Here's how the part is built. I have some questions about the finished solid (model axes, mm). Face numbers are marked on the shaded views. Give positions to 0.01 mm unless a question says otherwise; leave off trailing zeros. Order: outer loops, then holes, each group sorted by start corner. A loop starts at its lowest first (then second) coordinate and runs counter-clockwise, first axis right, second up.
from build123d import *

# Parameters (mm, degrees)
EXTRUDE_1_DEPTH     = 4
SKETCH_2_W          = 15
SKETCH_2_H          = 13.3866
CUT_EXTRUDE_1_DEPTH = 121.93395925
SKETCH_3_W          = 10
SKETCH_3_H          = 10
SKETCH_3_R          = 1.55
SKETCH_3_H_2        = 14.755
EXTRUDE_2_DEPTH     = 4
EXTRUDE_3_DEPTH     = 4
EXTRUDE_4_DEPTH     = 4
SKETCH_7_W          = 27.8
SKETCH_7_H          = 4
EXTRUDE_5_DEPTH     = 4
EXTRUDE_START       = -4
EXTRUDE_6_DEPTH     = 4
SKETCH_11_W         = 16.8
SKETCH_11_H         = 10.85
CUT_EXTRUDE_2_DEPTH = 133.52791749
CHAMFER_1_SIZE      = 2
CHAMFER_2_SIZE      = 2
SKETCH_12_W         = 12
SKETCH_12_H         = 8.55
SKETCH_12_R         = 1.25
EXTRUDE_7_DEPTH     = 4
EXTRUDE_START_2     = 4
SKETCH_13_R         = 1.25
SKETCH_13_W         = 4
SKETCH_13_H         = 8.709663749
EXTRUDE_8_DEPTH     = 4
SKETCH_14_R         = 1
CUT_EXTRUDE_3_DEPTH = 132.839329922
SKETCH_15_R         = 0.9
EXTRUDE_9_DEPTH     = 1
FILLET_1_R          = 0.9
CUT_EXTRUDE_START   = -1.7
SKETCH_16_R         = 1
CUT_EXTRUDE_4_DEPTH = 1.7
CUT_EXTRUDE_5_DEPTH = 132.839329922
SKETCH_19_W         = 5
SKETCH_19_H         = 38.5268
SKETCH_19_W_2       = 8.236887868
SKETCH_19_H_2       = 1.55
CUT_EXTRUDE_6_DEPTH = 132.839329922
EXTRUDE_12_DEPTH    = 23.28
CUT_EXTRUDE_7_REACH = 100.821
SKETCH_23_R         = 1.55
EXTRUDE_13_DEPTH    = 4
CUT_EXTRUDE_START_2 = -19.28
CUT_EXTRUDE_8_DEPTH = 19.48
SKETCH_26_W         = 10.1
SKETCH_26_H         = 2
EXTRUDE_14_DEPTH    = 3


# Read off the part's stored shape, not the designer's step: the extrude step
with BuildPart() as part:
    # Sketch 1 → Extrude 1 (new body)
    with BuildSketch(Plane.XY):
        with BuildLine():
            Line((-16.4, -7.25), (-16.4, 119.75))
            Line((-16.4, 119.75), (16.4, 119.75))
            Line((16.4, 119.75), (16.4, -7.25))
            ThreePointArc((16.4, -7.25), (15.038046533, -10.538046533), (11.75, -11.9))
            Line((11.75, -11.9), (-11.75, -11.9))
            ThreePointArc((-11.75, -11.9), (-15.038046533, -10.538046533), (-16.4, -7.25))
        make_face()
    extrude(amount=EXTRUDE_1_DEPTH)

    # Sketch 2 → Cut-Extrude 1 (cut, through all)
    with BuildSketch(Plane(origin=(0, 0, 0), x_dir=(-1, 0, 0), z_dir=(0, 0, -1))):
        with Locations((0, 110.2067)):
            Rectangle(SKETCH_2_W, SKETCH_2_H)
    extrude(amount=-CUT_EXTRUDE_1_DEPTH, mode=Mode.SUBTRACT)

    # Sketch 3 → Extrude 2 (add)
    # profile 1 of 2: a face of its own
    with BuildSketch(Plane(origin=(0, 119.75, 0), x_dir=(1, 0, 0), z_dir=(0, 1, 0))):
        with Locations((-18.9, 15.755)):
            Rectangle(SKETCH_3_W, SKETCH_3_H)
        with Locations(Location((-18.9, 15.755, 0), (0, 0, 270))):
            Circle(SKETCH_3_R, mode=Mode.SUBTRACT)
    # profile 2 of 2: a face of its own
    with BuildSketch(Plane(origin=(0, 119.75, 0), x_dir=(1, 0, 0), z_dir=(0, 1, 0))):
        with Locations((-18.9, 3.3775)):
            Rectangle(SKETCH_3_W, SKETCH_3_H_2)
    extrude_2 = extrude(amount=-EXTRUDE_2_DEPTH)

    # Mirror 1: Extrude 2 across plane
    add(extrude_2.mirror(Plane(origin=(0, 0, 0), x_dir=(0, 0, 1), z_dir=(1, 0, 0))))

    # Sketch 6 → Extrude 4 (add)
    with BuildSketch(Plane.XY.offset(4)):
        Polygon((-16.4, 115.75), (-23.9, 115.75), (-16.4, 108.25), align=None)
        Polygon((16.4, 115.75), (16.4, 108.25), (23.9, 115.75), align=None)
    extrude(amount=-EXTRUDE_4_DEPTH)

    # Sketch 7 → Extrude 5 (add)
    with BuildSketch(Plane(origin=(0, 119.75, 0), x_dir=(1, 0, 0), z_dir=(0, 1, 0))):
        with Locations((0, 18.755)):
            Rectangle(SKETCH_7_W, SKETCH_7_H)
    extrude(amount=-EXTRUDE_5_DEPTH)



with BuildPart() as body_2:
    # Sketch 5 → Extrude 3 (new body)
    with BuildSketch(Plane(origin=(0, 2.890336251, 0), x_dir=(1, 0, 0), z_dir=(0, 1, 0))):
        Polygon((50.795757056, 9.855), (46.095757056, 9.855), (32.240757056, -4), (39.311824868, -4), (51.095757056, 7.783932188), (51.095757056, 9.855), align=None)
        with BuildLine():
            Line((50.795757056, 18.755), (46.095757056, 18.755))
            Line((46.095757056, 18.755), (46.095757056, 9.855))
            Line((46.095757056, 9.855), (50.795757056, 9.855))
            Line((50.795757056, 9.855), (50.795757056, 15.105))
            Line((50.795757056, 15.105), (49.255691264, 15.105))
            ThreePointArc((49.255691264, 15.105), (47.495757056, 15.755), (49.255691264, 16.405))
            Line((49.255691264, 16.405), (50.795757056, 16.405))
            Line((50.795757056, 16.405), (50.795757056, 18.755))
        make_face()
        with BuildLine():
            Line((51.095757056, 18.755), (50.795757056, 18.755))
            Line((50.795757056, 18.755), (50.795757056, 16.405))
            Line((50.795757056, 16.405), (49.255691264, 16.405))
            ThreePointArc((49.255691264, 16.405), (49.433822674, 16.10145764), (49.495757056, 15.755))
            ThreePointArc((49.495757056, 15.755), (49.433822674, 15.40854236), (49.255691264, 15.105))
            Line((49.255691264, 15.105), (50.795757056, 15.105))
            Line((50.795757056, 15.105), (50.795757056, 9.855))
            Line((50.795757056, 9.855), (51.095757056, 9.855))
            Line((51.095757056, 9.855), (51.095757056, 18.755))
        make_face()
    extrude(amount=EXTRUDE_3_DEPTH)


with BuildPart() as part_1:
    add(part.part)

    add(body_2.part)  # Extrude 6 merges body 2
    # Sketch 8 → Extrude 6 (add)
    with BuildSketch(Plane.XY.offset(4).offset(EXTRUDE_START)):
        with BuildLine():
            Line((26.521488617, -11.9), (39.311824868, 0.890336251))
            Line((39.311824868, 0.890336251), (39.311824868, 6.890336251))
            Line((39.311824868, 6.890336251), (16.4, 6.890336251))
            Line((16.4, 6.890336251), (16.4, -7.25))
            ThreePointArc((16.4, -7.25), (15.038046533, -10.538046533), (11.75, -11.9))
            Line((11.75, -11.9), (26.521488617, -11.9))
        make_face()
    extrude(amount=EXTRUDE_6_DEPTH)

    # Sketch 11 → Cut-Extrude 2 (cut, through all)
    with BuildSketch(Plane.XY.offset(4)):
        with Locations((0, 1.525)):
            Rectangle(SKETCH_11_W, SKETCH_11_H)
        with Locations((0, 22.975)):
            Rectangle(SKETCH_11_W, SKETCH_11_H)
    extrude(amount=-CUT_EXTRUDE_2_DEPTH, mode=Mode.SUBTRACT)

    # Chamfer 1
    chamfer_1_edges = [part_1.edges().sort_by_distance(p)[0] for p in [
        (39.311824868, 2.890336251, 2),
    ]]
    chamfer(chamfer_1_edges, length=CHAMFER_1_SIZE - 0.0001)  # a hair under: the kernel refuses the full size

    # Chamfer 2
    chamfer_2_edges = [part_1.edges().sort_by_distance(p)[0] for p in [
        (38.776240962, 2.890336251, 0),
    ]]
    chamfer(chamfer_2_edges, length=CHAMFER_2_SIZE - 0.0001)  # a hair under: the kernel refuses the full size

    # Sketch 12 → Extrude 7 (add)
    with BuildSketch(Plane.ZY.offset(16.4)):
        with Locations((-2, 13.325)):
            Rectangle(SKETCH_12_W, SKETCH_12_H)
        with Locations((-4, 12.25)):
            Circle(SKETCH_12_R, mode=Mode.SUBTRACT)
    extrude(amount=EXTRUDE_7_DEPTH)

    # Sketch 13 → Extrude 8 (add)
    # profile 1 of 2: a face of its own
    with BuildSketch(Plane(origin=(16.4, 0, 0), x_dir=(0, 0, -1), z_dir=(1, 0, 0)).offset(EXTRUDE_START_2)):
        Polygon((8, 9.890336251), (8, 15.6), (0, 15.6), (0, 6.890336251), (5, 6.890336251), align=None)
        with Locations(Location((4, 12.25, 0), (0, 0, 180))):
            Circle(SKETCH_13_R, mode=Mode.SUBTRACT)
    # profile 2 of 2: a face of its own
    with BuildSketch(Plane(origin=(16.4, 0, 0), x_dir=(0, 0, -1), z_dir=(1, 0, 0)).offset(EXTRUDE_START_2)):
        with Locations((-2, 11.245168126)):
            Rectangle(SKETCH_13_W, SKETCH_13_H)
    extrude(amount=-EXTRUDE_8_DEPTH)

    # Sketch 14 → Cut-Extrude 3 (cut, through all)
    with BuildSketch(Plane(origin=(0, 0, 0), x_dir=(-1, 0, 0), z_dir=(0, 0, -1))):
        with Locations((-5, 62.6)):
            Circle(SKETCH_14_R)
        with Locations((-5, 99)):
            Circle(SKETCH_14_R)
    extrude(amount=-CUT_EXTRUDE_3_DEPTH, mode=Mode.SUBTRACT)

    # Sketch 15 → Extrude 9 (add)
    with BuildSketch(Plane(origin=(0, 0, 0), x_dir=(-1, 0, 0), z_dir=(0, 0, -1))):
        with Locations(Location((-5, 94.35, 0), (0, 0, 180))):
            Circle(SKETCH_15_R)
        with Locations(Location((-5, 57.98, 0), (0, 0, 180))):
            Circle(SKETCH_15_R)
    extrude(amount=EXTRUDE_9_DEPTH)

    # Fillet 1
    fillet_1_edges = [part_1.edges().sort_by_distance(p)[0] for p in [
        (4.1, 94.35, -1),
        (4.1, 57.98, -1),
    ]]
    fillet(fillet_1_edges, radius=FILLET_1_R)

    # Sketch 16 → Cut-Extrude 4 (cut)
    # profile 1 of 2: a face of its own
    with BuildSketch(Plane.XY.offset(4).offset(CUT_EXTRUDE_START)):
        Polygon((7.05, 61.416431948), (7.05, 63.783568052), (5, 64.967136104), (2.95, 63.783568052), (2.95, 61.416431948), (5, 60.232863896), align=None)
        with Locations(Location((5, 62.6, 0), (0, 0, 180))):
            Circle(SKETCH_16_R, mode=Mode.SUBTRACT)
    # profile 2 of 2: a face of its own
    with BuildSketch(Plane.XY.offset(4).offset(CUT_EXTRUDE_START)):
        Polygon((2.95, 97.816431948), (5, 96.632863896), (7.05, 97.816431948), (7.05, 100.183568052), (5, 101.367136104), (2.95, 100.183568052), align=None)
        with Locations(Location((5, 99, 0), (0, 0, 180))):
            Circle(SKETCH_16_R, mode=Mode.SUBTRACT)
    extrude(amount=CUT_EXTRUDE_4_DEPTH, mode=Mode.SUBTRACT)

    # Sketch 17 → Cut-Extrude 5 (cut, symmetric)
    with BuildSketch(Plane(origin=(0, 0, 0), x_dir=(-1, 0, 0), z_dir=(0, 0, -1))):
        Polygon((-12.5, 104.35), (-16.4, 108.25), (-16.4, 40.0866), (-12.5, 43.9866), align=None)
    cut_extrude_5 = extrude(amount=CUT_EXTRUDE_5_DEPTH, both=True, mode=Mode.SUBTRACT)

    # Mirror 2: Cut-Extrude 5 across plane
    add(cut_extrude_5.mirror(Plane(origin=(0, 0, 0), x_dir=(0, 0, 1), z_dir=(1, 0, 0))), mode=Mode.SUBTRACT)

    # Sketch 19 → Cut-Extrude 6 (cut, through all)
    with BuildSketch(Plane(origin=(0, 0, 0), x_dir=(-1, 0, 0), z_dir=(0, 0, -1))):
        with Locations((2, 74.25)):
            Rectangle(SKETCH_19_W, SKETCH_19_H)
        with Locations((0, 47.675)):
            Rectangle(SKETCH_19_W_2, SKETCH_19_H_2)
    extrude(amount=-CUT_EXTRUDE_6_DEPTH, mode=Mode.SUBTRACT)

    # Sketch 22 → Extrude 12 (add)
    with BuildSketch(Plane.XY.offset(4)):
        with BuildLine():
            Line((16.4, 32.719535971), (16.4, 31.75))
            Line((16.4, 31.75), (22.425, 31.75))
            Line((22.425, 31.75), (22.425, 37.75))
            Line((22.425, 37.75), (11.75, 37.75))
            Line((11.75, 37.75), (11.75, 36.5))
            ThreePointArc((11.75, 36.5), (14.746431556, 35.435633993), (16.4, 32.719535971))
        make_face()
    extrude_12 = extrude(amount=-EXTRUDE_12_DEPTH)

    # Sketch 23 → Cut-Extrude 7 (cut, up to next)
    with BuildSketch(Plane(origin=(0, 37.75, 0), x_dir=(1, 0, 0), z_dir=(0, 1, 0)), mode=Mode.PRIVATE) as cut_extrude_7_sk1:
        with Locations(Location((18.9, 15.755, 0), (0, 0, 270))):
            Circle(SKETCH_23_R)
    cut_extrude_7_tool1 = extrude(cut_extrude_7_sk1.sketch, amount=-CUT_EXTRUDE_7_REACH, mode=Mode.PRIVATE) & part_1.part
    # Sketch 23 → Cut-Extrude 7 (cut, up to next)
    with BuildSketch(Plane(origin=(0, 37.75, 0), x_dir=(1, 0, 0), z_dir=(0, 1, 0)), mode=Mode.PRIVATE) as cut_extrude_7_sk2:
        with BuildLine():
            ThreePointArc((18.9, 19.28), (21.392551404, 18.247551403), (22.425, 15.754999999))
            Line((22.425, 15.754999999), (22.425, 19.28))
            Line((22.425, 19.28), (18.9, 19.28))
        make_face()
    cut_extrude_7_tool2 = extrude(cut_extrude_7_sk2.sketch, amount=-CUT_EXTRUDE_7_REACH, mode=Mode.PRIVATE) & part_1.part
    cut_extrude_7_1 = cut_extrude_7_tool1.solids().sort_by_distance((18.9, 37.75, -15.755))[0]
    add(cut_extrude_7_1, mode=Mode.SUBTRACT)
    cut_extrude_7_2 = cut_extrude_7_tool2.solids().sort_by_distance((21.637628, 37.75, -18.492628))[0]
    add(cut_extrude_7_2, mode=Mode.SUBTRACT)
    cut_extrude_7 = cut_extrude_7_1 + cut_extrude_7_2  # Cut-Extrude 7 as one shape, for the pattern or mirror that repeats it

    # Sketch 24 → Extrude 13 (add)
    with BuildSketch(Plane.XY.offset(4)):
        Polygon((16.4, 40.0866), (18.7366, 37.75), (18.7366, 31.75), (16.4, 29.4134), align=None)
    extrude_13 = extrude(amount=-EXTRUDE_13_DEPTH)

    # Mirror 3: Extrude 12, Cut-Extrude 7, Extrude 13 across plane
    add(extrude_12.mirror(Plane(origin=(0, 0, 0), x_dir=(0, 0, 1), z_dir=(1, 0, 0))))
    add(cut_extrude_7.mirror(Plane(origin=(0, 0, 0), x_dir=(0, 0, 1), z_dir=(1, 0, 0))), mode=Mode.SUBTRACT)
    add(extrude_13.mirror(Plane(origin=(0, 0, 0), x_dir=(0, 0, 1), z_dir=(1, 0, 0))))

    # Cut-Extrude 8 outline → Cut-Extrude 8 (cut)
    with BuildSketch(Plane.XY.offset(CUT_EXTRUDE_START_2)):
        with BuildLine():
            ThreePointArc((-16.4, 31.75), (-16.318817794, 32.615103442), (-16.078105821, 33.45))
            Line((-16.078105821, 33.45), (-22.425, 33.45))
            Line((-22.425, 33.45), (-22.425, 31.75))
            Line((-22.425, 31.75), (-16.4, 31.75))
        make_face()
    extrude(amount=CUT_EXTRUDE_8_DEPTH, mode=Mode.SUBTRACT)

    # Sketch 26 → Extrude 14 (add, symmetric)
    with BuildSketch(Plane(origin=(0, 0, 0), x_dir=(0, 0, -1), z_dir=(1, 0, 0))):
        with Locations((1.05, -12.9)):
            Rectangle(SKETCH_26_W, SKETCH_26_H)
        Polygon((8.1, -11.9), (8.1, -13.9), (6.1, -13.9), (6.1, -11.9), (6.1, -10.9), (7.1, -10.9), align=None)
    extrude(amount=EXTRUDE_14_DEPTH, both=True)


solid = part_1.part
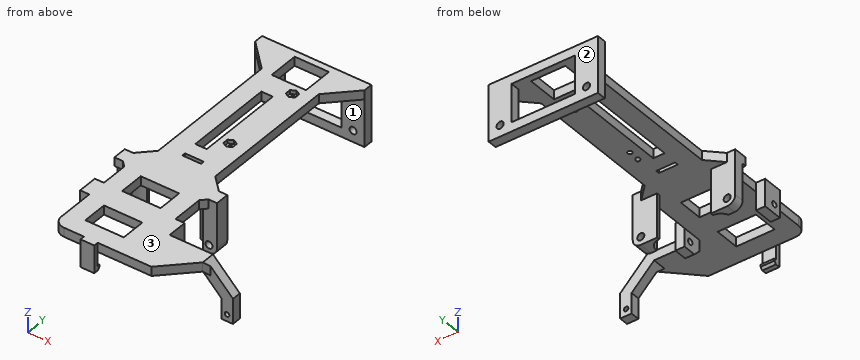
Q1. If we section it at C-C on y = 39: List the corners of the cut face in (x, z) for me, plus the area to 3 significant figures.
Filled sheet:
outline: (-17.49, 0) - (17.49, 0) - (17.49, 4) - (-17.49, 4) - close
area: 140 mm2
Q2. Thinking about a two-plate mould opening in Y: for the marked faces 1, 2 and 3, which applies, released by +Y, released by -Y, zero draft, split by the parting line, or undercut?
Filled sheet:
face 1: undercut
face 2: released by +Y
face 3: zero draft
Q3. If we section it at B-B on y = 24: List the corners of the cut face in (x, z) for me.
Filled sheet:
outline: (-16.4, 0) - (-8.4, 0) - (-8.4, 4) - (-16.4, 4) - close; (8.4, 0) - (16.4, 0) - (16.4, 4) - (8.4, 4) - close
Q4. I'm going to push flat-ended pins straight in: P1, Ø2.5, axis at x = 5, y = 62.6, coming from the -Z side; P2, Ø0.8, axis at y = 99, z = 2.5, coming from the +X side; P3, Ø1.8, axis at x = 18.5, z = -10, coming from the -Y side. Where does each tip first touch, or does it pass through?
Filled sheet:
P1: stops at z = 0
P2: stops at x = 12.5
P3: stops at y = 31.75
Q5. I need wall thicknesses on L1, parallel to Y at x = -19, z = -4; L2, parallel to Y at x = -6.5, z = 2; L3, parallel to Y at x = 17, z = -15. Which ranges of each line are inside material? Lowest first, please.
Filled sheet:
L1: y = 9.05 to 11, 13.5 to 17.6, 33.45 to 37.75, 115.75 to 119.75
L2: y = -11.9 to -3.9, 6.95 to 17.55, 28.4 to 103.51, 116.9 to 119.75
L3: y = 31.75 to 37.75, 115.75 to 119.75
Q6. If we section it at A-A on z = -12.75: List the corners of the cut face in (x, y) for me (3 decimals), plus the area to 3 significant figures.
Filled sheet:
outline: (-23.9, 115.75) - (-13.9, 115.75) - (-13.9, 119.75) - (-23.9, 119.75) - close; (-22.425, 33.45) - (-16.185, 33.45) arc R4.75 cw to (-11.75, 36.5) - (-11.75, 37.75) - (-22.425, 37.75) - close; (11.75, 36.5) arc R4.75 cw to (16.4, 32.72) - (16.4, 31.75) - (22.425, 31.75) - (22.425, 37.75) - (11.75, 37.75) - close; (13.9, 115.75) - (23.9, 115.75) - (23.9, 119.75) - (13.9, 119.75) - close; (46.096, 2.89) - (51.096, 2.89) - (51.096, 6.89) - (46.096, 6.89) - close
area: 182 mm2
